Build history of the part. All positions in model axes, mm. Face numbers are marked on the shaded views. A direction names the side the tool comes from. Coordinates: 2 decimals unless noted, no trailing zeros. Loops run counter-clockwise (first coordinate to the right, second up) from the corner with the lowest first, then second, coordinate; pieces in that order, holes last. Notation, with made-up numbers: (-23, 5) - (7, 5) arc R30 ccw to (7, 39) - close; hole circle Ø1 at (49, -7). An arc over 180 degrees is marked (long way). One line per item, written item: value.
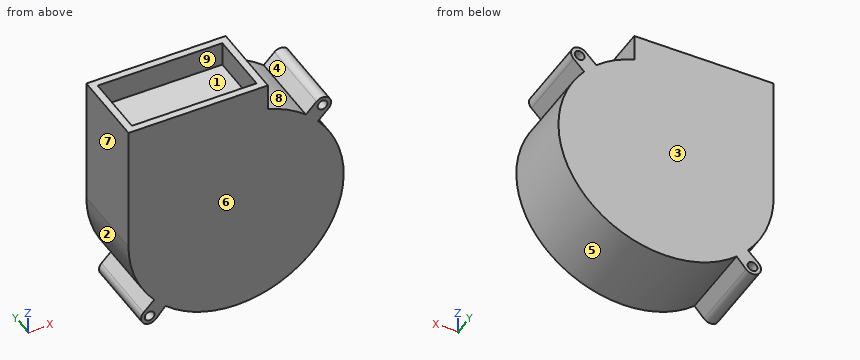
```python
from build123d import *

# Parameters (mm, degrees)
CROQUIS1_R              = 2
SALIENTE_EXTRUIR1_DEPTH = 32
CROQUIS2_W              = 51
CROQUIS2_H              = 26
CORTAR_EXTRUIR1_DEPTH   = 10


with BuildPart() as part:
    # Croquis1 → Saliente-Extruir1 (new body)
    with BuildSketch(Plane(origin=(0, 0, 0), x_dir=(1, 0, 0), z_dir=(0, 1, 0))):
        with BuildLine():
            Line((-37.830212793, 32.880465325), (-33.488983426, 28.539235958))
            ThreePointArc((-33.488983426, 28.539235958), (-41.28871075, 15.206655274), (-44, 0))
            Line((-44, 0), (-44, -53.035699114))
            Line((-44, -53.035699114), (13, -53.035699114))
            Line((13, -53.035699114), (13, -42.035699114))
            ThreePointArc((13, -42.035699114), (21.204683875, -38.553357594), (28.539235958, -33.488983426))
            Line((28.539235958, -33.488983426), (32.880465325, -37.830212793))
            ThreePointArc((32.880465325, -37.830212793), (37.830212793, -37.830212793), (37.830212793, -32.880465325))
            Line((37.830212793, -32.880465325), (33.488983426, -28.539235958))
            ThreePointArc((33.488983426, -28.539235958), (30.963432731, 31.261251311), (-28.858489769, 33.214267541))
            Line((-28.858489769, 33.214267541), (-32.71329505, 37.650900745))
            ThreePointArc((-32.71329505, 37.650900745), (-37.742020856, 37.915368356), (-37.830212793, 32.880465325))
        make_face()
        with Locations(Location((-35.355339059, 35.355339059, 0), (0, 0, 270))):
            Circle(CROQUIS1_R, mode=Mode.SUBTRACT)
        with Locations(Location((35.355339059, -35.355339059, 0), (0, 0, 270))):
            Circle(CROQUIS1_R, mode=Mode.SUBTRACT)
    extrude(amount=SALIENTE_EXTRUIR1_DEPTH)

    # Croquis2 → Cortar-Extruir1 (cut)
    with BuildSketch(Plane.XY.offset(53.035699114)):
        with Locations((-15.5, 16)):
            Rectangle(CROQUIS2_W, CROQUIS2_H)
    extrude(amount=-CORTAR_EXTRUIR1_DEPTH, mode=Mode.SUBTRACT)


solid = part.part
```
Item 1: Cut at A-A, the plane y = 26. Write the cut outline in (x, z).
Check result:
outline: (-44, 0) arc R44 ccw to (-33.49, -28.54) - (-37.83, -32.88) arc R3.5 ccw (long way) to (-32.71, -37.65) - (-28.86, -33.21) arc R44 ccw to (33.49, 28.54) - (37.83, 32.88) arc R3.5 ccw to (32.88, 37.83) - (28.54, 33.49) arc R44 ccw to (13, 42.04) - (13, 53.04) - (10, 53.04) - (10, 43.04) - (-41, 43.04) - (-41, 53.04) - (-44, 53.04) - close; hole circle Ø4 at (-35.36, -35.36); hole circle Ø4 at (35.36, 35.36)
Item 2: Probe probe 1 along X at (y, z) = (28.5, 44.5); probe 2 along Z at (x, y) = (-36, 20); probe 3 along Z at (x, y) = (-28.5, 19.5). List the from-to ranges inside material, lowest first. Write a range as from..to.
Check result:
probe 1: x = -44..-41, 10..13
probe 2: z = -38.8..-37.25, -33.46..-31.05, -25.3..43.04
probe 3: z = -33.52..43.04
Item 3: Tool access for the marked faces 1, 2, 3, 4 and 5: list every direction of +Z, -Z, +X, -X, +Y, -Y with a clear straight run to the whole face (end or side of a thin tool).
Check result:
face 1: +Z
face 2: -X, +Y, -Y
face 3: +Z, -Z, +X, -X, +Y
face 4: +Z, +Y, -Y
face 5: +Y, -Y
Item 4: Cut at D-D, the plane z = -24. Write the cut outline in (x, y).
Check result:
outline: (-36.88, 0) - (36.88, 0) - (36.88, 32) - (-36.88, 32) - close
Item 5: Drop flat-ended pins along their axis: P1, Ø3, axis at x = 31, y = 12.5, coming from the +Z side; P2, Ø5, axis at y = 7.5, z = -5.5, coming from the +X side; P3, Ø12, axis at y = 8.5, z = -16.5, coming from the +X side. Give the stop position or say it passes through.
Check result:
P1: stops at z = 37.45
P2: stops at x = 43.9
P3: stops at x = 42.73
Item 6: Pull direction X, two halves, no side cores. Call the marked faces 6, 7, 8 and 9: released by +X, released by -X, zero draft, split by the parting line, or undercut.
Check result:
face 6: zero draft
face 7: released by -X
face 8: undercut
face 9: undercut
Item 7: Cut at B-B, the plane z = 35. Write the cut outline in (x, y).
Check result:
outline: (-44, 0) - (26.66, 0) - (26.66, 32) - (-44, 32) - close; (30.05, 0) - (33.39, 0) - (33.39, 32) - (30.05, 32) - close; (37.32, 0) - (38.84, 0) - (38.84, 32) - (37.32, 32) - close
Item 8: Cut at C-C, the plane z = 14. Write the cut outline in (x, y), then the cut area to 3 significant figures.
Check result:
outline: (-44, 0) - (41.71, 0) - (41.71, 32) - (-44, 32) - close
area: 2,740 mm^2
